Source: CAD feature listing. Evaluate the final solid. Frame: model axes, mm. A direction names the side the tool comes from. Give positions to 0.01 mm unless a question says otherwise; leave off trailing zeros. Order: outer loops, then holes, each group sorted by start corner. A loop starts at its lowest first (then second) coordinate and runs counter-clockwise, first axis right, second up. Notation, with made-up numbers: (25.25, 52) - (52.25, 52) arc R19 cw to (52.25, 63) - close; hole circle Ø9 at (28, 50.25). An arc over 180 degrees is marked (long way). Write each question's results on one line, items separated by ' | '. Start each with the question number.
Item 1: Section C-C on z = 22. Output: boundary loops of the cut face in (x, y), and give its area (3 significant figures).
Item 2: Mould query, pull axis X, two halves, no side actions, for faces 4 (the flat face through (32, -3, -19.05)), 5 (the flat face through (19.05, -3, 22)), 6 (the flat face through (73, -3, -12.7)). Classes: released by +X, released by -X, zero draft, split by the parting line, or undercut.
Item 3: Contact query for flat-ended pins moving along their axis: pin 1 Ø1.9 at (y, z) = (-4, 16.5) entering from -X; pin 2 Ø1.9 at (x, y) = (-72.5, -2.5) entering from +Z; pin 3 Ø3 at (y, z) = (-4, 22.5) entering from +X. Output: stop coordinate, or through.
Item 4: Section B-B on x = -38.5. Output: boundary loops of the cut face in (y, z), and give its area (3 significant figures).
Item 5: Section A-A on y = -4.75. Output: boundary loops of the cut face in (x, z), and give its area (3 significant figures).
Item 6: Line query: line 1 along X through (y, z) = (-2.5, -20); line 2 along Z through (x, y) = (-35, -2.25); line 3 along Z through (x, y) = (60, -4.75). Output: solid intervals per line, ascending.
Item 7: Set-up query: faces 1 (the flat face through (69.85, -3, -19)), 2 (the flat face through (-41, -3, 19.05)), 3 (the flat face through (-44.45, -3, -22)). Return all of +Z, -Z, +X, -X, +Y, -Y with unobstructed straight access to the full face (end or side cutting, diameter ignored); none if empty.
```python
from build123d import *

# Parameters (mm, degrees)
F1_DEPTH = 6.35


with BuildPart() as f1:
    # F0 (on Front) → F1 (new body)
    with BuildSketch(Plane.XZ):
        Polygon((-69.85, 12.7), (-76.2, 12.7), (-76.2, 6.35), (-76.2, 0), (-76.2, -6.35), (-76.2, -12.7), (-69.85, -12.7), (-69.85, -19.05), (-69.85, -25.4), (-63.5, -25.4), (-57.15, -25.4), (-50.8, -25.4), (-44.45, -25.4), (-44.45, -19.05), (-38.1, -19.05), (-31.75, -19.05), (-25.4, -19.05), (-19.05, -19.05), (-19.05, -25.4), (-12.7, -25.4), (-6.35, -25.4), (0, -25.4), (6.35, -25.4), (12.7, -25.4), (19.05, -25.4), (19.05, -19.05), (25.4, -19.05), (31.75, -19.05), (38.1, -19.05), (44.45, -19.05), (44.45, -25.4), (50.8, -25.4), (57.15, -25.4), (63.5, -25.4), (69.85, -25.4), (69.85, -19.05), (69.85, -12.7), (76.2, -12.7), (76.2, -6.35), (76.2, 0), (76.2, 6.35), (76.2, 12.7), (69.85, 12.7), (69.85, 19.05), (63.5, 19.05), (57.15, 19.05), (50.8, 19.05), (44.45, 19.05), (38.1, 19.05), (31.75, 19.05), (25.4, 19.05), (19.05, 19.05), (19.05, 25.4), (12.7, 25.4), (6.35, 25.4), (0, 25.4), (-6.35, 25.4), (-12.7, 25.4), (-12.7, 19.05), (-19.05, 19.05), (-25.4, 19.05), (-31.75, 19.05), (-38.1, 19.05), (-44.45, 19.05), (-50.8, 19.05), (-57.15, 19.05), (-69.85, 19.05), align=None)
    extrude(amount=F1_DEPTH)


solid = f1.part
```
Evaluation:
1) outline: (-12.7, -6.35) - (19.05, -6.35) - (19.05, 0) - (-12.7, 0) - close | area: 202 mm^2
2) face 4: undercut | face 5: released by +X | face 6: zero draft
3) pin 1: stops at x = -69.85 | pin 2: stops at z = 12.7 | pin 3: stops at x = 19.05
4) outline: (-6.35, -19.05) - (0, -19.05) - (0, 19.05) - (-6.35, 19.05) - close | area: 242 mm^2
5) outline: (-76.2, -12.7) - (-69.85, -12.7) - (-69.85, -25.4) - (-44.45, -25.4) - (-44.45, -19.05) - (-19.05, -19.05) - (-19.05, -25.4) - (19.05, -25.4) - (19.05, -19.05) - (44.45, -19.05) - (44.45, -25.4) - (69.85, -25.4) - (69.85, -12.7) - (76.2, -12.7) - (76.2, 12.7) - (69.85, 12.7) - (69.85, 19.05) - (19.05, 19.05) - (19.05, 25.4) - (-12.7, 25.4) - (-12.7, 19.05) - (-69.85, 19.05) - (-69.85, 12.7) - (-76.2, 12.7) - close | area: 6,410 mm^2
6) line 1: x = -69.85 to -44.45, -19.05 to 19.05, 44.45 to 69.85 | line 2: z = -19.05 to 19.05 | line 3: z = -25.4 to 19.05
7) face 1: -Z, +X, +Y, -Y | face 2: +Z, -X, +Y, -Y | face 3: -Z, +Y, -Y
